Design review of the part shown in the three views and the two pictorial views. Dimensions are in mm from the part's minimum x, y and z. Give positions to 0.01 mm unless a question says otherwise; leave off trailing zeros. Order: outer loops, then holes, each group sorted by start corner. A loop starts at its lowest first (then second) coordinate and runs counter-clockwise, first axis right, second up.
Item 1: Consider section C-C (x = 101). Give the boundary of the cut face in (y, z).
Item 2: Consider section B-B (z = 1.9). Give the number of separate pieces and of enclosed holes in the cut face, plus the area to 3 significant figures.
Item 3: For probe 1 along Y at (x, z) = (41.5, 1.05); probe 2 along Y at (x, z) = (101, 2.35); probe 3 along X at (y, z) = (8, 1.8), list the stretches that pass through material, from the lowest coordinate up.
Item 4: Consider section A-A (x = 23.5). Give the boundary of the cut face in (y, z), plus the area to 3 significant figures.
Item 5: For P1, Ø1.5, axis at x = 133.5, z = 2.5, coming from the -Y side; P2, Ø2.5, axis at x = 121, y = 24, coming from the +Z side, all flat-tipped, find the tip position at first contact; note any pin that passes through.
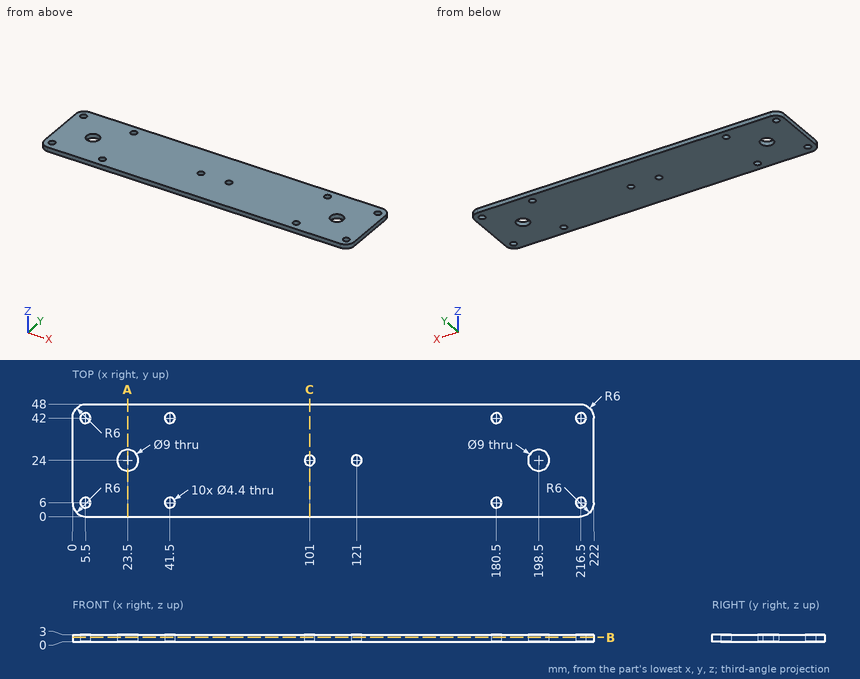
Resolved:
1. outline: (0, 0) - (21.8, 0) - (21.8, 3) - (0, 3) - close; (26.2, 0) - (48, 0) - (48, 3) - (26.2, 3) - close
2. separate pieces: 1
2. enclosed holes: 12
2. area: 10,300 mm2
3. probe 1: y = 0 to 3.8, 8.2 to 39.8, 44.2 to 48
3. probe 2: y = 0 to 21.8, 26.2 to 48
3. probe 3: x = 0 to 4.58, 6.42 to 40.58, 42.42 to 179.58, 181.42 to 215.58, 217.42 to 222
4. outline: (0, 0) - (19.5, 0) - (19.5, 3) - (0, 3) - close; (28.5, 0) - (48, 0) - (48, 3) - (28.5, 3) - close
4. area: 117 mm2
5. P1: stops at y = 0
5. P2: passes through
